Check sheet for the modelled part. Datum: model origin and axes. Units: mm. Face numbers are marked on the shaded views. A direction names the side the tool comes from. Give positions to 0.01 mm unless a question says otherwise; leave off trailing zeros. Loops run counter-clockwise (first coordinate to the right, second up) from the corner with the lowest first, then second, coordinate; pieces in that order, holes last. Notation, with made-up numbers: M 79,53 L 118,53 A7 cw 118,66 Z; hole C -39,74.5 d7. An arc over 180 degrees is marked long. One line per question, with ' | ' between items. Start each with the question number.
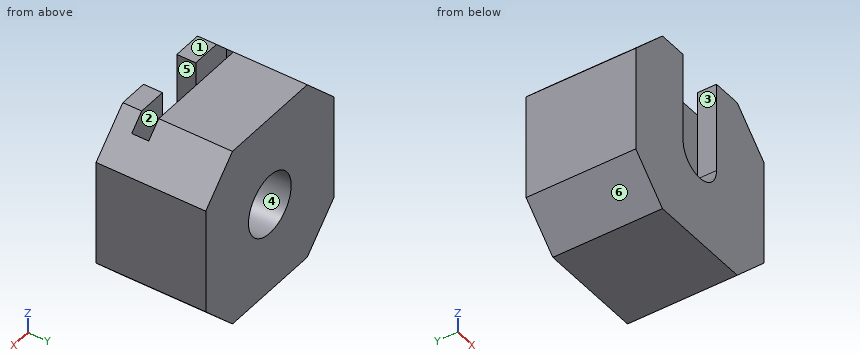
from build123d import *

# Parameters (mm, degrees)
SKETCH1_W           = 24.384
SKETCH1_H           = 24.384
BOSS_EXTRUDE1_DEPTH = 12.192
SKETCH2_W           = 24.384
SKETCH2_H           = 24.384
SKETCH2_R           = 3.175
BOSS_EXTRUDE2_DEPTH = 2.54
SKETCH3_W           = 6.35
SKETCH3_H           = 12.192
CUT_EXTRUDE1_DEPTH  = 2.54
CUT_EXTRUDE2_DEPTH  = 2.286
SKETCH5_W           = 24.384
SKETCH5_H           = 24.384
SKETCH5_R           = 4.064
BOSS_EXTRUDE3_DEPTH = 9.906
CHAMFER1_SIZE       = 5.08


with BuildPart() as part:
    # Sketch1 → Boss-Extrude1 (new body)
    with BuildSketch(Plane(origin=(0, 0, 0), x_dir=(1, 0, 0), z_dir=(0, 1, 0))):
        Rectangle(SKETCH1_W, SKETCH1_H)
        Polygon((-6.096, 9.017), (6.096, 9.017), (9.017, 6.096), (9.017, -6.096), (6.096, -9.017), (-6.096, -9.017), (-9.017, -6.096), (-9.017, 6.096), align=None, mode=Mode.SUBTRACT)
    extrude(amount=BOSS_EXTRUDE1_DEPTH)

    # Sketch2 → Boss-Extrude2 (add)
    with BuildSketch(Plane.XZ):
        Rectangle(SKETCH2_W, SKETCH2_H)
        with Locations(Location((0, 0, 0), (0, 0, 270))):
            Circle(SKETCH2_R, mode=Mode.SUBTRACT)
    extrude(amount=BOSS_EXTRUDE2_DEPTH)

    # Sketch3 → Cut-Extrude1 (cut)
    with BuildSketch(Plane.XZ.offset(2.54)):
        with Locations((0, 6.096)):
            Rectangle(SKETCH3_W, SKETCH3_H)
    extrude(amount=-CUT_EXTRUDE1_DEPTH, mode=Mode.SUBTRACT)

    # Sketch4 → Cut-Extrude2 (cut)
    with BuildSketch(Plane(origin=(0, 0, 0), x_dir=(1, 0, 0), z_dir=(0, 1, 0))):
        Polygon((-3.175, -6.096), (-9.017, -6.096), (-6.096, -9.017), (-3.175, -9.017), align=None)
        Polygon((-6.096, -9.017), (-9.017, -6.096), (-9.017, -12.192), (9.017, -12.192), (9.017, -6.096), (6.096, -9.017), (3.175, -9.017), (3.175, -6.096), (-3.175, -6.096), (-3.175, -9.017), align=None)
        Polygon((9.017, -6.096), (3.175, -6.096), (3.175, -9.017), (6.096, -9.017), align=None)
    extrude(amount=CUT_EXTRUDE2_DEPTH, mode=Mode.SUBTRACT)

    # Sketch5 → Boss-Extrude3 (add)
    with BuildSketch(Plane(origin=(0, 12.192, 0), x_dir=(1, 0, 0), z_dir=(0, 1, 0))):
        Rectangle(SKETCH5_W, SKETCH5_H)
        with Locations(Location((0, 0, 0), (0, 0, 270))):
            Circle(SKETCH5_R, mode=Mode.SUBTRACT)
    extrude(amount=-BOSS_EXTRUDE3_DEPTH)

    # Chamfer1
    # the kernel refuses this chamfer: 5.08 mm, written as the material it takes off along each edge
    with BuildSketch(Plane(origin=(12.192, 25.256149579, -12.192), x_dir=(0.027495876610586254, -5.537865568379339e-15, 0.9996219169112968), z_dir=(0, -1, 0)), Plane(origin=(12.192, -15.604149579, 12.192), x_dir=(0.027495876610586268, 0, -0.9996219169112968), z_dir=(0, 1, 0))) as chamfer1_piece_1:
        Polygon((CHAMFER1_SIZE * 0.999621916911, CHAMFER1_SIZE * 0.0274958766106), (-CHAMFER1_SIZE * 0.0274958766106, CHAMFER1_SIZE * 0.999621916911), (0, 0), align=None)
    extrude(amount=40.860299158, mode=Mode.SUBTRACT)
    with BuildSketch(Plane(origin=(-12.192, 25.256149579, -12.192), x_dir=(-0.027495876610586265, -3.4921279629514554e-15, 0.9996219169112968), z_dir=(0, -1, 0)), Plane(origin=(-12.192, -15.604149579, 12.192), x_dir=(-0.027495876610586275, 0, -0.9996219169112968), z_dir=(0, 1, 0))) as chamfer1_piece_2:
        Polygon((CHAMFER1_SIZE * 0.999621916911, -CHAMFER1_SIZE * 0.0274958766106), (-CHAMFER1_SIZE * 0.0274958766106, -CHAMFER1_SIZE * 0.999621916911), (0, 0), align=None)
    extrude(amount=40.860299158, mode=Mode.SUBTRACT)


solid = part.part
Q1. Cross-section at D-D (x = 5). Record the cut outline in (y, z).
Q2. Access from +Z, -Z, +X, -X, +Y, -Y to the whole of each face (thin tool, end or side, straight path). Record for the marked faces 1, 2 and 3.
Q3. Cross-section at B-B (y = 6). Record the cut outline in (x, z), and give its area (3 significant figures).
Q4. Cross-section at A-A (x = 0). Record the cut outline in (y, z) (3 decimals).
Q5. Depth check by flat-ended pin: P1, Ø13, axis at x = 0, z = 0, coming from the -Y side; P2, Ø1.1, axis at x = 0, y = 1, coming from the +Z side; P3, Ø0.8, axis at y = -1.5, z = 8.5, coming from the +X side; P4, Ø2, axis at x = 8.5, y = 5, coming from the +Z side. Enter the tip coordinate at first touch or a pass-through.
Q6. Material ranges on probe 1 along Y at (x, z) = (7.5, 2.75); probe 2 along X at (y, z) = (-1.5, 4.5) (3 decimals); probe 3 along X at (y, z) = (8.5, 0), recorded low to high. Write a range as from..to.
Q7. Cross-section at C-C (z = 5). Record the cut outline in (x, y) (3 decimals).
Q8. Draft check along Z on the marked faces 4, 5 and 6. Enter one of: released by +Z, released by -Z, zero draft, split by the parting line, or undercut.
Solved:
1) outline: M -2.54,-12.19 L 12.19,-12.19 L 12.19,12.19 L 2.29,12.19 L 2.29,-9.02 L 0,-9.02 L 0,12.19 L -2.54,12.19 Z
2) face 1: +Z, +X, -X, +Y, -Y | face 2: +Z | face 3: +Z, -Y
3) outline: M -12.19,-7.11 L -7.11,-12.19 L 7.11,-12.19 L 12.19,-7.11 L 12.19,7.11 L 7.11,12.19 L -7.11,12.19 L -12.19,7.11 Z; hole C 0,0 d8.13 | area: 491 mm²
4) outline: M -2.54,-12.192 L 12.192,-12.192 L 12.192,-4.064 L 2.286,-4.064 L 2.286,-9.017 L 0,-9.017 L 0,-3.175 L -2.54,-3.175 Z; M 2.286,4.064 L 12.192,4.064 L 12.192,12.192 L 2.286,12.192 Z
5) P1: stops at y = -2.54 | P2: stops at z = -9.02 | P3: stops at x = 11.2 | P4: stops at z = 11.8
6) probe 1: y = -2.54..0, 2.29..12.19 | probe 2: x = -12.192..-3.175, 3.175..12.192 | probe 3: x = -12.19..-4.06, 4.06..12.19
7) outline: M -12.192,-2.54 L -3.175,-2.54 L -3.175,0 L -9.017,0 L -9.017,2.286 L 9.017,2.286 L 9.017,0 L 3.175,0 L 3.175,-2.54 L 12.192,-2.54 L 12.192,12.192 L -12.192,12.192 Z
8) face 4: undercut | face 5: zero draft | face 6: released by -Z
